Autodesk Inventor part; units mm, degrees
ref_plane "YZ Plane" through (0, 0, 0) normal (1, 0, 0) x (0, 1, 0)
ref_plane "XZ Plane" through (0, 0, 0) normal (0, 1, 0) x (-1, 0, 0)
ref_plane "XY Plane" through (0, 0, 0) normal (0, 0, 1) x (1, 0, 0)
sketch "Sketch1" plane through (0, 0, 0) normal (0, 1, 0) x (-1, 0, 0)
  line L0 (0, 0) -> (6.35, 0)
  line L1 (6.35, 0) -> (6.35, -6.35)
  line L2 (6.35, -6.35) -> (0, -6.35)
  line L3 (0, -6.35) -> (0, 0)
  line L4 (7.62, -7.62) -> (7.62, 1.27)
  line L5 (7.62, 1.27) -> (-1.27, 1.27)
  line L6 (-1.27, 1.27) -> (-1.27, -7.62)
  line L7 (-1.27, -7.62) -> (7.62, -7.62)
  dimension "d0" = 6.35
  dimension "d1" = 6.35
  dimension "d2" = 1.27
extrude "Extrusion1" add sketch "Sketch1" along normal blind 5.08 contours L0 L1 L2 L3
extrude "Extrusion2" add sketch "Sketch1" along normal blind 2.54
properties part number "LED"
The listing builds one solid part. Answer for the finished solid, in the listing's coordinates (mm). A direction names the side the tool comes from. Coordinates: 2 decimals unless noted, no trailing zeros. Order: outer loops, then holes, each group sorted by start corner. A loop starts at its lowest first (then second) coordinate and runs counter-clockwise, first axis right, second up. Notation, with made-up numbers: (-2.75, -6.5) -> (18.25, -6.5) arc R23 ccw to (18.25, 9.5) -> close; hole circle Ø2 at (-15.5, -6). An arc over 180 degrees is marked (long way). Answer in a Markdown table with one row per item. Add a question column.
Item 1: Find section D-D (z = 0.25). Write down the section's boundary in (x, y).
Item 2: Find section B-B (z = -4). Write down the section's boundary in (x, y).
Item 3: Which of the six approach directions +Z, -Z, +X, -X, +Y, -Y give full straight-line access (tool end or side, diameter ignored) to faces 1 (the face through (-3, 4, 0)), 2 (the face through (-6.35, 4, -3)), 3 (the face through (-7.62, 1, -3)), 4 (the face through (-3, 4, -6.35)), 5 (the face through (0, 4, -3))?
Item 4: Find section C-C (y = 4.3). Write down the section's boundary in (x, z).
Item 5: Find section A-A (x = -4.5). Write down the section's boundary in (y, z), then the cut area to 3 significant figures.
Item 6: Find the intervals of material crossed by L1, parallel to X at y = 2.6, z = -5; L2, parallel to Y at x = -3.5, z = -7, in increasing order. Write a range as from..to.
Item 7: Each of these flat-tipped pins is pushed along its axis until it touches: P1, Ø2, axis at y = 4.5, z = -4, coming from the -X side; P2, Ø2, axis at y = 4, z = -4.5, coming from the +X side. Where does it stop, or does it pass through?
Result set:
| question | item | result |
|---|---|---|
| 1 | outline | (-7.62, 0) -> (1.27, 0) -> (1.27, 2.54) -> (-7.62, 2.54) -> close |
| 2 | outline | (-7.62, 0) -> (1.27, 0) -> (1.27, 2.54) -> (0, 2.54) -> (0, 5.08) -> (-6.35, 5.08) -> (-6.35, 2.54) -> (-7.62, 2.54) -> close |
| 3 | face 1 | +Z, +X, -X, +Y |
| 3 | face 2 | +Z, -Z, -X, +Y |
| 3 | face 3 | +Z, -Z, -X, +Y, -Y |
| 3 | face 4 | -Z, +X, -X, +Y |
| 3 | face 5 | +Z, -Z, +X, +Y |
| 4 | outline | (-6.35, -6.35) -> (0, -6.35) -> (0, 0) -> (-6.35, 0) -> close |
| 5 | outline | (0, -7.62) -> (2.54, -7.62) -> (2.54, -6.35) -> (5.08, -6.35) -> (5.08, 0) -> (2.54, 0) -> (2.54, 1.27) -> (0, 1.27) -> close |
| 5 | area | 38.7 mm² |
| 6 | L1 | x = -6.35..0 |
| 6 | L2 | y = 0..2.54 |
| 7 | P1 | stops at x = -6.35 |
| 7 | P2 | stops at x = 0 |
